```python
from build123d import *

# Parameters (mm, degrees)
SKETCH1_R           = 2
SKETCH1_W           = 6.35
SKETCH1_H           = 12.7
SKETCH1_H_2         = 6.35
SKETCH1_W_2         = 38.1
SKETCH1_H_3         = 69.85
BOSS_EXTRUDE1_DEPTH = 6.35


with BuildPart() as part:
    # Sketch1 → Boss-Extrude1 (new body)
    with BuildSketch(Plane(origin=(0, 0, 0), x_dir=(1, 0, 0), z_dir=(0, 1, 0))):
        Polygon((12.7, 117.475), (0, 89.958333333), (0, 76.2), (19.05, 76.2), (19.05, 88.9), (25.4, 88.9), (25.4, 76.2), (38.1, 76.2), (38.1, 96.8375), (31.75, 117.475), align=None)
        with Locations((22.225, 95.25)):
            Circle(SKETCH1_R, mode=Mode.SUBTRACT)
        with Locations((22.225, 107.95)):
            Rectangle(SKETCH1_W, SKETCH1_H, mode=Mode.SUBTRACT)
        Polygon((0, 76.2), (-6.35, 76.2), (-6.35, -9.525), (12.7, -15.875), (38.1, -15.875), (44.45, -9.525), (44.45, 76.2), (38.1, 76.2), (25.4, 76.2), (19.05, 76.2), align=None)
        with Locations((15.875, -6.35)):
            Rectangle(SKETCH1_W, SKETCH1_H_2, mode=Mode.SUBTRACT)
        with Locations((34.925, -6.35)):
            Rectangle(SKETCH1_W, SKETCH1_H_2, mode=Mode.SUBTRACT)
        with Locations((19.05, 34.925)):
            Rectangle(SKETCH1_W_2, SKETCH1_H_3, mode=Mode.SUBTRACT)
        Polygon((0, 89.958333333), (-6.35, 76.2), (0, 76.2), align=None)
        Polygon((44.45, 76.2), (38.1, 96.8375), (38.1, 76.2), align=None)
    extrude(amount=BOSS_EXTRUDE1_DEPTH)


solid = part.part
```
The listing builds one solid part. Answer for the finished solid, in the listing's coordinates (mm). A direction names the side the tool comes from. Coordinates: 2 decimals unless noted, no trailing zeros. Write each loop counter-clockwise with the first axis right and the second up, starting at its lowest first coordinate (ties: lowest second). Pieces come first, ordered by that corner, then holes. Notation, with made-up numbers: (48.5, 22.5) -> (90.5, 22.5) arc R19 ccw to (90.5, 52.5) -> close; hole circle Ø1 at (-10, 6.5). An arc over 180 degrees is marked (long way). Write each question's results on one line, items separated by ' | '. Start each with the question number.
1) Straight lines are drawn through the part: probe 1 along Z at (x, y) = (17, 2) (3 decimals); probe 2 along X at (y, z) = (4.5, -60.5). For each, find the intervals that lie inside material, in ascending order.
2) For a pull along X with two mould halves and no side action, classify faces 1 (the flat face through (41.231, 3.131, 12.744)), 2 (the flat face through (22, 3, -117.475)), 3 (the flat face through (35, 3, 9.525)) as +X half, -X half, draft (parallel to the pull), parting line (faces both ways), or undercut.
3) A tool of negligible diameter and unlimited length cuts with its end or side. For faces 4 (the flat face through (0, 3, -34)), 5 (the flat face through (-6.35, 3, -34)), from which of +Z, -Z, +X, -X, +Y, -Y can it reach the whole face along a straight path? Write none if from no direction.
4) Flat-ended cylindrical pins translate along their axes: pin 1 Ø1.5 at (y, z) = (4.5, -93.5) entering from -X; pin 2 Ø5 at (x, z) = (22.225, -95.25) entering from +Y; pin 3 Ø3 at (y, z) = (2, -82) entering from -X; pin 4 Ø5 at (x, z) = (16, -4) entering from -Y. Find the tip coordinate at first contact, or state that the pin passes through.
5) A cutting plane is placed at C-C (y = 3.25). Count the separate pieces of the cut face and the enclosed holes in it, then the cut area to 3 significant figures.
6) A cutting plane is placed at A-A (z = -64.5). Determine the outline of the cut face in (x, y), then the cut area to 3 significant figures.
7) A cutting plane is placed at B-B (x = 21.5). Determine the outline of the cut face in (y, z) (3 decimals), then the cut area to 3 significant figures.
Values follow:
1) probe 1: -117.475 to -69.85, 0 to 3.175, 9.525 to 15.875 | probe 2: -6.35 to 0, 38.1 to 44.45
2) face 1: +X half | face 2: draft | face 3: undercut
3) face 4: +Y, -Y | face 5: +Z, -Z, -X, +Y, -Y
4) pin 1: x = 1.29 | pin 2: y = 6.35 | pin 3: x = -4.37 | pin 4: through
5) separate pieces: 1 | enclosed holes: 6 | area: 3,120 mm²
6) outline: (-6.35, 0) -> (0, 0) -> (0, 6.35) -> (-6.35, 6.35) -> close; (38.1, 0) -> (44.45, 0) -> (44.45, 6.35) -> (38.1, 6.35) -> close | area: 80.6 mm²
7) outline: (0, -117.475) -> (6.35, -117.475) -> (6.35, -114.3) -> (0, -114.3) -> close; (0, -101.6) -> (6.35, -101.6) -> (6.35, -97.114) -> (0, -97.114) -> close; (0, -93.386) -> (6.35, -93.386) -> (6.35, -88.9) -> (0, -88.9) -> close; (0, -76.2) -> (6.35, -76.2) -> (6.35, -69.85) -> (0, -69.85) -> close; (0, 0) -> (6.35, 0) -> (6.35, 15.875) -> (0, 15.875) -> close | area: 218 mm²
